Model file for the job. Use its own axes, mm. A direction names the side the tool comes from. Give positions to 0.01 mm unless a question says otherwise; leave off trailing zeros. Write each loop counter-clockwise with the first axis right and the second up, starting at its lowest first coordinate (ties: lowest second). Pieces come first, ordered by that corner, then holes. Notation, with made-up numbers: M 50.5,3 L 70.5,3 A13 ccw 70.5,22 Z; hole C -28.75,38 d8. An arc over 180 degrees is marked long. Answer as a JSON object with one key per item and string values. Group by question number.
```python
from build123d import *

# Parameters (mm, degrees)
F0_W          = 40
F0_H          = 40
F1_DEPTH      = 2
F2_W          = 2
F2_H          = 39
F3_DEPTH      = 20
F3_DEPTH_BACK = 20
F5_D          = 3


with BuildPart() as f1:
    # F0 (on Top) → F1 (new body)
    with BuildSketch(Plane.XY):
        Rectangle(F0_W, F0_H)
    extrude(amount=F1_DEPTH)

    # F2 (on Right) → F3 (join, two sides)
    with BuildSketch(Plane.YZ) as f3_sk:
        with Locations((-19, -19.5)):
            Rectangle(F2_W, F2_H)
    extrude(amount=F3_DEPTH)
    extrude(f3_sk.sketch, amount=-F3_DEPTH_BACK)

    # F5 (through all)
    with Locations(Plane.XY.offset(2)):
        with Locations((-17, -16), (17, -16)):
            Hole(F5_D / 2)


solid = f1.part
```
Q1. Slice it at C-C, the plane x = 2.5. Write the cut outline in (y, z).
Q2. Drop flat-ended pins along their axis: P1, Ø2.5, axis at x = -17, y = -16, coming from the -Z side; P2, Ø1.5, axis at x = 16, z = -12.5, coming from the +Y side; P3, Ø19, axis at x = 6.5, y = 4, coming from the -Z side. Give the stop position or say it passes through.
Q3. Slice it at D-D, the plane z = -21.5. Write the cut outline in (x, y).
Q4. Wall check: L1, parallel to Y at x = -17, z = 1; L2, parallel to Z at x = -9, y = 17; L3, parallel to Y at x = -4.5, z = -15. Give the ranges that are in metal, low to high.
Q5. 3-axis set-ups, long thin cutter, end or side, ignore diameter. For faces 4 (the flat face through (0, -19, -39)), 5 (the flat face through (0, 1, 0)): which of +Z, -Z, +X, -X, +Y, -Y reach the whole face in a straight line?
Q6. Two-plate mould, pull along X, no slides. Class faces 1 (the flat face through (20, -19, -9)), 2 (the cylindrical face through (-15.5, -15.93, 0.99)), 3 (the flat face through (0, 20, 1)): +X half, -X half, draft (parallel to the pull), parting line (faces both ways), or undercut.
Q7. Slice it at A-A, the plane x = -17. Write the cut outline in (y, z).
Q8. Slice it at B-B, the plane y = -16. Write the cut outline in (x, z).
Solved:
{
 "1": {"outline": "M -20,-39 L -18,-39 L -18,0 L 20,0 L 20,2 L -20,2 Z"},
 "2": {"P1": "passes through", "P2": "stops at y = -18", "P3": "stops at z = 0"},
 "3": {"outline": "M -20,-20 L 20,-20 L 20,-18 L -20,-18 Z"},
 "4": {"L1": "y = -20 to -17.5, -14.5 to 20", "L2": "z = 0 to 2", "L3": "y = -20 to -18"},
 "5": {"face 4": "-Z, +X, -X, +Y, -Y", "face 5": "-Z, +X, -X, +Y"},
 "6": {"face 1": "+X half", "face 2": "undercut", "face 3": "draft"},
 "7": {"outline": "M -20,-39 L -18,-39 L -18,0 L -17.5,0 L -17.5,2 L -20,2 Z; M -14.5,0 L 20,0 L 20,2 L -14.5,2 Z"},
 "8": {"outline": "M -20,0 L -18.5,0 L -18.5,2 L -20,2 Z; M -15.5,0 L 15.5,0 L 15.5,2 L -15.5,2 Z; M 18.5,0 L 20,0 L 20,2 L 18.5,2 Z"}
}
